Design review of the part built by this model. Coordinates are the model's own, in mm. A direction names the side the tool comes from. Coordinates: 2 decimals unless noted, no trailing zeros. Loops run counter-clockwise (first coordinate to the right, second up) from the corner with the lowest first, then second, coordinate; pieces in that order, holes last. Notation, with made-up numbers: (-34.5, 39) - (-10.5, 39) arc R19 cw to (-10.5, 61) - close; hole circle Ø4 at (21, 69). An arc over 180 degrees is marked (long way). One line per question, with ' | ' between items.
from build123d import *

# Parameters (mm, degrees)
BOSS_EXTRUDE2_DEPTH = 30
SKETCH2_W           = 80
SKETCH2_H           = 80
BOSS_EXTRUDE3_DEPTH = 55
CUT_EXTRUDE1_DEPTH  = 70
SKETCH4_R           = 15
BOSS_EXTRUDE4_DEPTH = 5
SKETCH6_R           = 10
CUT_EXTRUDE2_DEPTH  = 91
SKETCH7_R           = 30
BOSS_EXTRUDE5_DEPTH = 15
SKETCH8_R           = 10
CUT_EXTRUDE3_DEPTH  = 46
CUT_EXTRUDE4_DEPTH  = 15
SKETCH11_W          = 30
SKETCH11_H          = 20
CUT_EXTRUDE5_DEPTH  = 91
SKETCH12_R          = 15
BOSS_EXTRUDE6_DEPTH = 20
CUT_EXTRUDE6_REACH  = 112
SKETCH13_R          = 10
SKETCH14_R          = 15
BOSS_EXTRUDE7_DEPTH = 10
SKETCH15_R          = 10
CUT_EXTRUDE7_DEPTH  = 15
SKETCH16_R          = 5
CUT_EXTRUDE8_DEPTH  = 26
SKETCH17_W          = 60
SKETCH17_H          = 10
CUT_EXTRUDE9_DEPTH  = 15
RIB1_REACH          = 62
SKETCH18_WALL_W     = 172
SKETCH18_WALL_H     = 10


with BuildPart() as part:
    # Sketch1 → Boss-Extrude2 (new body)
    with BuildSketch(Plane(origin=(0, 0, 0), x_dir=(1, 0, 0), z_dir=(0, 1, 0))):
        with BuildLine():
            Line((130, 30), (130, -30))
            ThreePointArc((130, -30), (110, -50), (90, -30))
            Line((90, -30), (40, -30))
            Line((40, -30), (40, -40))
            Line((40, -40), (-40, -40))
            Line((-40, -40), (-104.747935056, -29.621902584))
            ThreePointArc((-104.747935056, -29.621902584), (-130, 0), (-104.747935056, 29.621902584))
            Line((-104.747935056, 29.621902584), (-40, 40))
            Line((-40, 40), (40, 40))
            Line((40, 40), (40, 30))
            Line((40, 30), (90, 30))
            ThreePointArc((90, 30), (110, 50), (130, 30))
        make_face()
    extrude(amount=BOSS_EXTRUDE2_DEPTH)

    # Sketch2 → Boss-Extrude3 (add)
    with BuildSketch(Plane(origin=(0, 30, 0), x_dir=(1, 0, 0), z_dir=(0, 1, 0))):
        Rectangle(SKETCH2_W, SKETCH2_H)
    extrude(amount=BOSS_EXTRUDE3_DEPTH)

    # Sketch3 → Cut-Extrude1 (cut)
    with BuildSketch(Plane.XZ):
        with BuildLine():
            Line((-20, -30), (20, -30))
            ThreePointArc((20, -30), (27.071067812, -27.071067812), (30, -20))
            Line((30, -20), (30, 20))
            ThreePointArc((30, 20), (27.071067812, 27.071067812), (20, 30))
            Line((20, 30), (-20, 30))
            ThreePointArc((-20, 30), (-27.071067812, 27.071067812), (-30, 20))
            Line((-30, 20), (-30, -20))
            ThreePointArc((-30, -20), (-27.071067812, -27.071067812), (-20, -30))
        make_face()
    extrude(amount=-CUT_EXTRUDE1_DEPTH, mode=Mode.SUBTRACT)

    # Sketch4 → Boss-Extrude4 (add)
    with BuildSketch(Plane(origin=(0, 85, 0), x_dir=(1, 0, 0), z_dir=(0, 1, 0))):
        with Locations(Location((0, 0, 0), (0, 0, 270))):  # turned: the seam where the file's is
            Circle(SKETCH4_R)
    extrude(amount=BOSS_EXTRUDE4_DEPTH)

    # Sketch6 → Cut-Extrude2 (cut, through all)
    with BuildSketch(Plane(origin=(0, 90, 0), x_dir=(1, 0, 0), z_dir=(0, 1, 0))):
        with Locations(Location((0, 0, 0), (0, 0, 270))):  # turned: the seam where the file's is
            Circle(SKETCH6_R)
    extrude(amount=-CUT_EXTRUDE2_DEPTH, mode=Mode.SUBTRACT)

    # Sketch7 → Boss-Extrude5 (add)
    with BuildSketch(Plane(origin=(0, 30, 0), x_dir=(1, 0, 0), z_dir=(0, 1, 0))):
        with Locations(Location((-100, 0, 0), (0, 0, 99.10617604))):  # turned: the seam where the file's is
            Circle(SKETCH7_R)
    extrude(amount=BOSS_EXTRUDE5_DEPTH)

    # Sketch8 → Cut-Extrude3 (cut, through all)
    with BuildSketch(Plane(origin=(0, 45, 0), x_dir=(1, 0, 0), z_dir=(0, 1, 0))):
        with Locations(Location((-100, 0, 0), (0, 0, 270))):  # turned: the seam where the file's is
            Circle(SKETCH8_R)
    extrude(amount=-CUT_EXTRUDE3_DEPTH, mode=Mode.SUBTRACT)

    # Sketch9 → Cut-Extrude4 (cut)
    with BuildSketch(Plane.XZ):
        with BuildLine():
            Line((-50, 28.269512751), (-50, -28.269512751))
            Line((-50, -28.269512751), (-103.165290037, -19.747935056))
            ThreePointArc((-103.165290037, -19.747935056), (-120, 0), (-103.165290037, 19.747935056))
            Line((-103.165290037, 19.747935056), (-50, 28.269512751))
        make_face()
    extrude(amount=-CUT_EXTRUDE4_DEPTH, mode=Mode.SUBTRACT)

    # Sketch11 → Cut-Extrude5 (cut, through all)
    with BuildSketch(Plane.XY.offset(40)):
        with Locations((0, 10)):
            Rectangle(SKETCH11_W, SKETCH11_H)
    extrude(amount=-CUT_EXTRUDE5_DEPTH, mode=Mode.SUBTRACT)

    # Sketch12 → Boss-Extrude6 (add)
    with BuildSketch(Plane.XY.offset(40)):
        with Locations(Location((0, 55, 0), (0, 0, 180))):  # turned: the seam where the file's is
            Circle(SKETCH12_R)
    extrude(amount=BOSS_EXTRUDE6_DEPTH)

    # Sketch13 → Cut-Extrude6 (cut, up to next)
    with BuildSketch(Plane.XY.offset(60), mode=Mode.PRIVATE) as cut_extrude6_sk1:
        with Locations((0, 55)):
            Circle(SKETCH13_R)
    cut_extrude6_tool1 = extrude(cut_extrude6_sk1.sketch, amount=-CUT_EXTRUDE6_REACH, mode=Mode.PRIVATE) & part.part
    add(cut_extrude6_tool1.solids().sort_by_distance((0, 55, 60))[0], mode=Mode.SUBTRACT)

    # Sketch14 → Boss-Extrude7 (add)
    with BuildSketch(Plane(origin=(0, 30, 0), x_dir=(1, 0, 0), z_dir=(0, 1, 0))):
        with Locations(Location((110, -30, 0), (0, 0, 270))):  # turned: the seam where the file's is
            Circle(SKETCH14_R)
        with Locations(Location((110, 30, 0), (0, 0, 270))):  # turned: the seam where the file's is
            Circle(SKETCH14_R)
    extrude(amount=BOSS_EXTRUDE7_DEPTH)

    # Sketch15 → Cut-Extrude7 (cut)
    with BuildSketch(Plane(origin=(0, 40, 0), x_dir=(1, 0, 0), z_dir=(0, 1, 0))):
        with Locations(Location((110, -30, 0), (0, 0, 270))):  # turned: the seam where the file's is
            Circle(SKETCH15_R)
        with Locations(Location((110, 30, 0), (0, 0, 270))):  # turned: the seam where the file's is
            Circle(SKETCH15_R)
    extrude(amount=-CUT_EXTRUDE7_DEPTH, mode=Mode.SUBTRACT)

    # Sketch16 → Cut-Extrude8 (cut, through all)
    with BuildSketch(Plane(origin=(0, 25, 0), x_dir=(1, 0, 0), z_dir=(0, 1, 0))):
        with Locations(Location((110, -30, 0), (0, 0, 270))):  # turned: the seam where the file's is
            Circle(SKETCH16_R)
        with Locations(Location((110, 30, 0), (0, 0, 270))):  # turned: the seam where the file's is
            Circle(SKETCH16_R)
    extrude(amount=-CUT_EXTRUDE8_DEPTH, mode=Mode.SUBTRACT)

    # Sketch17 → Cut-Extrude9 (cut)
    with BuildSketch(Plane(origin=(0, 30, 0), x_dir=(1, 0, 0), z_dir=(0, 1, 0))):
        with Locations((100, 0)):
            Rectangle(SKETCH17_W, SKETCH17_H)
    extrude(amount=-CUT_EXTRUDE9_DEPTH, mode=Mode.SUBTRACT)

    # Sketch18 wall → Rib1 (add, up to next)
    with BuildSketch(Plane(origin=(-55, 65, 0), x_dir=(0.6, 0.8, 0), z_dir=(-0.8, 0.6, 0)), mode=Mode.PRIVATE) as rib1_sk1:
        Rectangle(SKETCH18_WALL_W, SKETCH18_WALL_H)
    rib1_tool1 = extrude(rib1_sk1.sketch, amount=-RIB1_REACH, mode=Mode.PRIVATE) - part.part
    add(rib1_tool1.solids().sort_by_distance((-55, 65, 0))[0])


solid = part.part
Q1. Take a section at C-C (y = 79). Give the boundary of the cut face in (x, z).
Returned:
outline: (-44.5, -5) - (-40, -5) - (-40, -40) - (40, -40) - (40, 40) - (-40, 40) - (-40, 5) - (-44.5, 5) - close; hole circle Ø20 at (0, 0)
Q2. To check wall thickness, follow line 1 along Z through (x, y) = (15.5, 57.5); line 2 along X through (y, z) = (64, 36). State the ranges of each line that lie inside material, in increasing order.
Returned:
line 1: z = -40 to -30, 30 to 40 | line 2: x = -40 to -4.36, 4.36 to 40
Q3. Tool access review of faces 1 (the flat face through (15, 10, 35)), 2 (the flat face through (100, 40, -27)), 3 (the flat face through (-102, 45, -13)), 4 (the flat face through (-40, 57, -22)), 5 (the flat face through (17, 85, -1)): name each direction out of +Z, -Z, +X, -X, +Y, -Y from which nothing blocks a thin tool from reaching the whole face with its end or side.
Returned:
face 1: +Z, -Z, -Y | face 2: +Z, -Z, +X, +Y | face 3: +Z, -Z, -X, +Y | face 4: -Z, +Y | face 5: +Y
Q4. Take a section at A-A (y = 37). Give the boundary of the cut face in (x, z).
Returned:
outline: (-70.42, -5) - (-40, -5) - (-40, -40) - (40, -40) - (40, 40) - (-40, 40) - (-40, 5) - (-70.42, 5) arc R30 ccw (long way) to start; circle Ø30 at (110, -30); circle Ø30 at (110, 30); hole circle Ø20 at (-100, 0); hole (-30, -20) arc R10 ccw to (-20, -30) - (20, -30) arc R10 ccw to (30, -20) - (30, 20) arc R10 ccw to (20, 30) - (-20, 30) arc R10 ccw to (-30, 20) - close; hole circle Ø20 at (110, -30); hole circle Ø20 at (110, 30)
Q5. Take a section at B-B (x = 110). State how many separate pieces and enclosed holes the cut face has, plus the area to 3 significant figures.
Returned:
separate pieces: 3 | enclosed holes: 0 | area: 2,350 mm²
Q6. For pin 1 (10 mm diameter, centred on x = 10.5, y = 29, fed in from +Z); pin 2 (7.5 mm diameter, centred on x = 103.5, y = 20.5, fed in from +Z); pin 3 (3 mm diameter, centred on y = 23.5, z = -11, fed in from -X); pin 4 (8 mm diameter, centred on x = 110, z = -30, fed in from +Y), all flat-tipped, find the tip position at first contact; note any pin that passes through.
Returned:
pin 1: stops at z = 40 | pin 2: stops at z = 49.81 | pin 3: stops at x = -128.46 | pin 4: passes through
Q7. Take a section at D-D (x = -100). Give the boundary of the cut face in (y, z), plus the area to 3 significant figures.
Returned:
outline: (0, -30.38) - (30, -30.38) - (30, -30) - (45, -30) - (45, -10) - (15, -10) - (15, -20.26) - (0, -20.26) - close; (0, 20.26) - (15, 20.26) - (15, 10) - (45, 10) - (45, 30) - (30, 30) - (30, 30.38) - (0, 30.38) - close | area: 1,520 mm²
Q8. Draft analysis for pull direction Z (two halves, no side actions). For faces 6 (the flat face through (0, 42, 30)), 7 (the flat face through (107, 40, 40)), 8 (the flat face through (-10, 58, 60)), state which applies: +Z half, -Z half, draft (parallel to the pull), parting line (faces both ways), or undercut.
Returned:
face 6: undercut | face 7: draft | face 8: +Z half
